Model file for the job. Use its own axes, mm. A direction names the side the tool comes from. Coordinates: 2 decimals unless noted, no trailing zeros. Order: outer loops, then holes, each group sorted by start corner. A loop starts at its lowest first (then second) coordinate and runs counter-clockwise, first axis right, second up. Notation, with made-up numbers: (63.5, -19) -> (100.5, -19) arc R21 cw to (100.5, 13) -> close; hole circle Ø10 at (-7, 44). An arc over 180 degrees is marked (long way). Write item = value, one per line. Start each with the question number.
Q1. Cut at B-B, the plane z = 45. List the corners of the cut face in (x, y), plus the area to 3 significant figures.
Q2. Mould opens along Z. For faces 1 (the face through (-141.15, -23.84, 11.04)), 2 (the face through (132.826, -45.885, 16.291)), 3 (the face through (-1, 0, -99)), 4 (the face through (33.718, -23.837, 136.207)) say: +Z half, -Z half, draft (parallel to the pull), parting line (faces both ways), or undercut.
Q3. Cut at A-A, the plane x = -132.5. List the corners of the cut face in (y, z).
Q4. Wall check: line 1 (X direction, y = -20, z = -99.5); line 2 (X direction, y = -39.5, z = 171); line 3 (Z direction, x = -161.5, y = -46). Give the ranges that are in metal, low to high. Write a range as from..to.
Q5. Flat gauge pins, fed straight in: pin 1 (4 mm diameter, centred on x = 68.5, y = -10, fed in from -Z); pin 2 (1 mm diameter, centred on y = -23.5, z = -37.5, fed in from +X); pin 3 (1.5 mm diameter, centred on y = -14.5, z = 102, fed in from +X). Where does each tip first touch, or does it go through?
Q6. 3-axis set-ups, long thin cutter, end or side, ignore diameter. For faces 5 (the face through (-107.34, -23.84, -90.37)), 6 (the face through (52.78, -23.84, -130.01)), 7 (the face through (-131.53, -45.885, 14.881)): which of +Z, -Z, +X, -X, +Y, -Y reach the whole face in a straight line?
from build123d import *

# Parameters (mm, degrees)
F1_DEPTH = 48.35
F2_SIZE  = 5
F3_SIZE  = 2


with BuildPart() as f1:
    # F0 (on Front) → F1 (new body)
    with BuildSketch(Plane.XZ):
        Polygon((3.3454659382, 184.4213456143), (0, 191.2), (-3.4042833476, 184.3021685259), (-0.0588174093, 177.5235141402), align=None)
        with BuildLine():
            Line((3.3454659382, 184.4213456143), (6.6341131163, 191.0848726173))
            ThreePointArc((6.6341131163, 191.0848726173), (3.3175559963, 191.1712159877), (0, 191.2))
            Line((0, 191.2), (3.3454659382, 184.4213456143))
        make_face()
        with BuildLine():
            Line((-3.4042833476, 184.3021685259), (0, 191.2))
            ThreePointArc((0, 191.2), (-3.3754006651, 191.1702034062), (-6.7497492858, 191.0808229116))
            Line((-6.7497492858, 191.0808229116), (-3.4042833476, 184.3021685259))
        make_face()
        Polygon((-3.4042833476, 184.3021685259), (-6.7497492858, 191.0808229116), (-60.2314095212, 82.7151430913), (-53.0235747303, 83.7625027933), align=None)
        Polygon((-0.0588174093, 177.5235141402), (-3.4042833476, 184.3021685259), (-53.0235747303, 83.7625027933), (-56.1922701192, 77.3420246622), (-49.5013382427, 77.3420246622), align=None)
        Polygon((52.9688284065, 83.8734309614), (3.3454659382, 184.4213456143), (-0.0588174093, 177.5235141402), (49.383703424, 77.3420246622), (56.1922701192, 77.3420246622), align=None)
        Polygon((60.054246696, 82.8438594182), (6.6341131163, 191.0848726173), (3.3454659382, 184.4213456143), (52.9688284065, 83.8734309614), align=None)
        Polygon((52.0811544326, 71.876391938), (58.2598817772, 70.9785703011), (56.1922701192, 77.3420246622), (49.383703424, 77.3420246622), align=None)
        Polygon((63.2776884086, 76.312453119), (60.054246696, 82.8438594182), (52.9688284065, 83.8734309614), (56.1922701192, 77.3420246622), align=None)
        Polygon((174.2297969358, 60.1901680357), (179.6428745321, 65.4666146204), (60.054246696, 82.8438594182), (63.2776884086, 76.312453119), align=None)
        Polygon((168.8167193396, 54.9137214509), (174.2297969358, 60.1901680357), (63.2776884086, 76.312453119), (56.1922701192, 77.3420246622), (58.2598817772, 70.9785703011), align=None)
        Polygon((96.1366412096, -24.458033873), (176.4289283194, 53.8076027397), (168.8167193396, 54.9137214509), (88.8170401417, -23.0666929402), (90.9210029578, -29.5420246622), align=None)
        Polygon((97.3469751481, -31.5148222116), (183.7825669636, 52.7390564976), (176.4289283194, 53.8076027397), (96.1366412096, -24.458033873), align=None)
        Polygon((176.4289283194, 53.8076027397), (181.8420059156, 59.0840493245), (174.2297969358, 60.1901680357), (168.8167193396, 54.9137214509), align=None)
        with BuildLine():
            Line((174.2297969358, 60.1901680357), (181.8420059156, 59.0840493245))
            ThreePointArc((181.8420059156, 59.0840493245), (180.7706115026, 62.2850384682), (179.6428745321, 65.4666146204))
            Line((179.6428745321, 65.4666146204), (174.2297969358, 60.1901680357))
        make_face()
        with BuildLine():
            Line((176.4289283194, 53.8076027397), (183.7825669636, 52.7390564976))
            ThreePointArc((183.7825669636, 52.7390564976), (182.8398118758, 55.9199713271), (181.8420059156, 59.0840493245))
            Line((181.8420059156, 59.0840493245), (176.4289283194, 53.8076027397))
        make_face()
        Polygon((85.5079253616, -33.4748557433), (90.9210029578, -29.5420246622), (88.8170401417, -23.0666929402), (84.4524727268, -27.3210946961), align=None)
        Polygon((92.1313368964, -36.5988130009), (97.3469751481, -31.5148222116), (96.1366412096, -24.458033873), (90.9210029578, -29.5420246622), align=None)
        Polygon((104.3932878305, -143.5849678348), (111.0842197069, -147.1025988913), (92.1313368964, -36.5988130009), (90.9210029578, -29.5420246622), (85.5079253616, -33.4748557433), align=None)
        Polygon((111.0842197069, -147.1025988913), (117.7751515833, -150.6202299478), (97.3469751481, -31.5148222116), (92.1313368964, -36.5988130009), align=None)
        Polygon((105.6936083619, -151.166418268), (112.3845402383, -154.6840493245), (111.0842197069, -147.1025988913), (104.3932878305, -143.5849678348), align=None)
        with BuildLine():
            ThreePointArc((112.3845402383, -154.6840493245), (115.0977827408, -152.6759326422), (117.7751515833, -150.6202299478))
            Line((117.7751515833, -150.6202299478), (111.0842197069, -147.1025988913))
            Line((111.0842197069, -147.1025988913), (112.3845402383, -154.6840493245))
        make_face()
        with BuildLine():
            ThreePointArc((106.9497598069, -158.4903431672), (109.6836622396, -156.6107730576), (112.3845402383, -154.6840493245))
            Line((112.3845402383, -154.6840493245), (105.6936083619, -151.166418268))
            Line((105.6936083619, -151.166418268), (106.9497598069, -158.4903431672))
        make_face()
        Polygon((0.1094926475, -102.3210906944), (106.9497598069, -158.4903431672), (105.6936083619, -151.166418268), (6.4468834252, -98.9893271929), align=None)
        Polygon((6.4468834252, -98.9893271929), (105.6936083619, -151.166418268), (104.3932878305, -143.5849678348), (5.5082461637, -91.5980249074), (0, -95.6), align=None)
        Polygon((-6.3373907777, -98.9317635015), (0.1094926475, -102.3210906944), (6.4468834252, -98.9893271929), (0, -95.6), align=None)
        Polygon((0, -95.6), (5.5082461637, -91.5980249074), (0.1133441465, -88.7617570701), (-5.4130775962, -91.6671689189), align=None)
        Polygon((-104.298119263, -143.6541118464), (-105.5759735432, -151.1045739839), (-6.3373907777, -98.9317635015), (0, -95.6), (-5.4130775962, -91.6671689189), align=None)
        Polygon((-105.5759735432, -151.1045739839), (-106.8538278234, -158.5550361215), (0.1094926475, -102.3210906944), (-6.3373907777, -98.9317635015), align=None)
        Polygon((-111.1066859581, -147.2335871869), (-112.3845402383, -154.6840493245), (-105.5759735432, -151.1045739839), (-104.298119263, -143.6541118464), align=None)
        with BuildLine():
            ThreePointArc((-117.6839803143, -150.6914754635), (-115.0515806012, -152.7107520811), (-112.3845402383, -154.6840493245))
            Line((-112.3845402383, -154.6840493245), (-111.1066859581, -147.2335871869))
            Line((-111.1066859581, -147.2335871869), (-117.6839803143, -150.6914754635))
        make_face()
        with BuildLine():
            ThreePointArc((-112.3845402383, -154.6840493245), (-109.636269739, -156.6439541052), (-106.8538278234, -158.5550361215))
            Line((-106.8538278234, -158.5550361215), (-105.5759735432, -151.1045739839))
            Line((-105.5759735432, -151.1045739839), (-112.3845402383, -154.6840493245))
        make_face()
        Polygon((-92.1522481313, -36.7207348557), (-111.1066859581, -147.2335871869), (-104.298119263, -143.6541118464), (-85.4127567941, -33.5439997549), (-90.9210029578, -29.5420246622), align=None)
        Polygon((-97.2793049704, -31.7230896035), (-117.6839803143, -150.6914754635), (-111.1066859581, -147.2335871869), (-92.1522481313, -36.7207348557), align=None)
        Polygon((-90.9210029578, -29.5420246622), (-85.4127567941, -33.5439997549), (-84.3824221918, -27.5366880744), (-88.8533912998, -23.1785703011), align=None)
        Polygon((-96.048059797, -24.54437941), (-97.2793049704, -31.7230896035), (-92.1522481313, -36.7207348557), (-90.9210029578, -29.5420246622), align=None)
        Polygon((-168.8530704977, 54.80184409), (-176.3337597519, 53.7148363136), (-96.048059797, -24.54437941), (-90.9210029578, -29.5420246622), (-88.8533912998, -23.1785703011), align=None)
        Polygon((-176.3337597519, 53.7148363136), (-183.8144490062, 52.6278285372), (-97.2793049704, -31.7230896035), (-96.048059797, -24.54437941), align=None)
        Polygon((-174.3613166614, 60.1710571009), (-181.8420059156, 59.0840493245), (-176.3337597519, 53.7148363136), (-168.8530704977, 54.80184409), align=None)
        with BuildLine():
            ThreePointArc((-181.8420059156, 59.0840493245), (-182.8567238392, 55.864644873), (-183.8144490062, 52.6278285372))
            Line((-183.8144490062, 52.6278285372), (-176.3337597519, 53.7148363136))
            Line((-176.3337597519, 53.7148363136), (-181.8420059156, 59.0840493245))
        make_face()
        with BuildLine():
            Line((-174.3613166614, 60.1710571009), (-179.6824595725, 65.3578895158))
            ThreePointArc((-179.6824595725, 65.3578895158), (-180.7894495105, 62.230337824), (-181.8420059156, 59.0840493245))
            Line((-181.8420059156, 59.0840493245), (-174.3613166614, 60.1710571009))
        make_face()
        Polygon((-60.2314095212, 82.7151430913), (-179.6824595725, 65.3578895158), (-174.3613166614, 60.1710571009), (-63.4001049101, 76.2946649602), align=None)
        Polygon((-63.4001049101, 76.2946649602), (-174.3613166614, 60.1710571009), (-168.8530704977, 54.80184409), (-58.2962329353, 70.8666929402), (-56.1922701192, 77.3420246622), align=None)
        Polygon((-53.0235747303, 83.7625027933), (-60.2314095212, 82.7151430913), (-63.4001049101, 76.2946649602), (-56.1922701192, 77.3420246622), align=None)
        Polygon((-52.2645491141, 71.7431479025), (-49.5013382427, 77.3420246622), (-56.1922701192, 77.3420246622), (-58.2962329353, 70.8666929402), align=None)
    extrude(amount=F1_DEPTH)

    # F2
    f2_edges = [f1.edges().sort_by_distance(p)[0] for p in [
        (-126.617746, -48.35, 13.632578),
        (-94.340271, -48.35, -85.5954),
        (-52.092388, -48.35, -116.207934),
        (52.253316, -48.35, -116.173362),
        (94.42288, -48.35, -85.453031),
        (126.634596, -48.35, 13.796313),
        (110.448937, -48.35, 63.395057),
        (26.011169, -48.35, 124.699953),
        (-26.161683, -48.35, 124.633331),
        (-110.55881, -48.35, 63.272496),
    ]]
    chamfer(f2_edges, length=F2_SIZE)

    # F3
    f3_edges = [f1.edges().sort_by_distance(p)[0] for p in [
        (-84.382422, -21.675, -27.536688),
        (-52.264549, -21.675, 71.743148),
        (0.113344, -21.675, -88.761757),
        (84.452473, -21.675, -27.321095),
        (52.081154, -21.675, 71.876392),
    ]]
    chamfer(f3_edges, length=F3_SIZE)


solid = f1.part
Here are the results:
q1.outline = (-175.99, -48.35) -> (-165.96, -48.35) -> (-158.8, -43.35) -> (-158.8, 0) -> (-175.99, 0) -> close; (158.65, -43.35) -> (165.81, -48.35) -> (175.84, -48.35) -> (175.84, 0) -> (158.65, 0) -> close
q1.area = 1,630 mm²
q2.face_1 = undercut
q2.face_2 = undercut
q2.face_3 = draft
q2.face_4 = +Z half
q3.outline = (-48.35, 2.61) -> (0, 2.61) -> (0, 19.37) -> (-43.35, 19.37) -> (-48.35, 12.38) -> close; (-48.35, 65.14) -> (-43.35, 60.08) -> (0, 60.08) -> (0, 72.21) -> (-48.35, 72.21) -> close
q4.line_1 = -108.9..-96.73, -20.31..20.54, 96.83..109.01
q4.line_2 = -16.66..-3.28, 3.16..16.55
q4.line_3 = 30.88..43.93, 58.55..68
q5.pin_1 = -139.33
q5.pin_2 = 98.46
q5.pin_3 = 50.97
q6.face_5 = -X, +Y, -Y
q6.face_6 = -Z, +Y, -Y
q6.face_7 = -Y
